Geometry check sheet. Reference: the model listing, model coordinates, mm. A direction names the side the tool comes from. Round coordinates to 2 decimals unless told otherwise and drop trailing zeros. Write each loop counter-clockwise with the first axis right and the second up, starting at its lowest first coordinate (ties: lowest second). Pieces come first, ordered by that corner, then holes.
Item 1: Draft check along Z on faces 4 (the face through (0, -11, -14)), 5 (the face through (23, 13, 3)), 6 (the face through (0.1, 14.5, 4.15)), 7 (the face through (-26, -8, -2)). Enter one of: pulls with the +Z half, pulls with the -Z half, needs draft (parallel to the pull), parting line crosses it, or undercut.
Item 2: Cross-section at A-A (z = -9). Enter the section's corners in (x, y) (3 decimals), then the cut area to 3 significant figures.
Item 3: Cross-section at C-C (x = 18). Enter the section's corners in (y, z).
Item 4: Access from +Z, -Z, +X, -X, +Y, -Y to the whole of each face (thin tool, end or side, straight path). Record for faces 1 (the face through (0.1, 14.5, 1.85)), 2 (the face through (0, -9, -9)), 3 (the face through (0, 11.6, 3)).
Item 5: Cross-section at B-B (y = -12). Enter the section's corners in (x, z) (3 decimals), then the cut area to 3 significant figures.
Item 6: Scan lines: probe 1 along Z at (x, y) = (19, -10.55) (3 decimals); probe 2 along Y at (x, z) = (-15, 1.5); probe 3 along Y at (x, z) = (-0.5, 1.5). Record each from-to range of solid material in increasing order.
Item 7: Cross-section at D-D (y = 2.75). Enter the section's corners in (x, z).
Item 8: Depth check by flat-ended pin: P1, Ø4, axis at y = 2.5, z = -2.5, coming from the +X side; P2, Ø6, axis at x = 6, y = 8.5, coming from the -Z side; P3, Ø1.8, axis at x = -15.5, z = 3, coming from the +Y side; P4, Ø1.5, axis at x = -0.5, z = 1.5, coming from the -Y side. Enter the tip coordinate at first touch or a pass-through.
from build123d import *

# Parameters (mm, degrees)
SKETCH_W        = 52
SKETCH_H        = 30
PAD_DEPTH       = 6
SKETCH001_R     = 6.15
POCKET_DEPTH    = 6
SKETCH002_W     = 30
SKETCH002_H     = 2.3
POCKET001_DEPTH = 2
SKETCH003_W     = 52
SKETCH003_H     = 2.3
POCKET002_DEPTH = 2
SKETCH004_W     = 30
SKETCH004_H     = 2.3
POCKET003_DEPTH = 2
SKETCH005_W     = 52
SKETCH005_H     = 6
PAD001_DEPTH    = 14
SKETCH006_W     = 19.5
SKETCH006_H     = 3.75
POCKET004_DEPTH = 26
CHAMFER_SIZE    = 4
SKETCH007_W     = 45
SKETCH007_H     = 2
PAD002_DEPTH    = 6
SKETCH008_R     = 1.875
POCKET005_DEPTH = 6


with BuildPart() as part:
    # Sketch → Pad (new body)
    with BuildSketch(Plane.XY):
        Rectangle(SKETCH_W, SKETCH_H)
    extrude(amount=PAD_DEPTH)

    # Sketch001 (on Face6 of Pad) → Pocket (cut)
    with BuildSketch(Plane.XY.offset(6)):
        with Locations((-16, 6)):
            Circle(SKETCH001_R)
        with Locations((0, 6)):
            Circle(SKETCH001_R)
        with Locations((16, 6)):
            Circle(SKETCH001_R)
    extrude(amount=-POCKET_DEPTH, mode=Mode.SUBTRACT)

    # Sketch002 (on Face3 of Pocket) → Pocket001 (cut)
    with BuildSketch(Plane.YZ.offset(26)):
        with Locations((0, 3)):
            Rectangle(SKETCH002_W, SKETCH002_H)
    extrude(amount=-POCKET001_DEPTH, mode=Mode.SUBTRACT)

    # Sketch003 (on Face1 of Pocket001) → Pocket002 (cut)
    with BuildSketch(Plane(origin=(0, 15, 0), x_dir=(-1, 0, 0), z_dir=(0, 1, 0))):
        with Locations((0, 3)):
            Rectangle(SKETCH003_W, SKETCH003_H)
    extrude(amount=-POCKET002_DEPTH, mode=Mode.SUBTRACT)

    # Sketch004 (on Face6 of Pocket002) → Pocket003 (cut)
    with BuildSketch(Plane(origin=(-26, 0, 0), x_dir=(0, -1, 0), z_dir=(-1, 0, 0))):
        with Locations((0, 3)):
            Rectangle(SKETCH004_W, SKETCH004_H)
    extrude(amount=-POCKET003_DEPTH, mode=Mode.SUBTRACT)

    # Sketch005 (on Face2 of Pocket003) → Pad001 (join)
    with BuildSketch(Plane(origin=(0, 0, 0), x_dir=(1, 0, 0), z_dir=(0, 0, -1))):
        with Locations((0, 12)):
            Rectangle(SKETCH005_W, SKETCH005_H)
    extrude(amount=PAD001_DEPTH)

    # Sketch006 (on Face19 of Pad001) → Pocket004 (cut)
    with BuildSketch(Plane.XY.offset(6)):
        with Locations((1.25, -13.125)):
            Rectangle(SKETCH006_W, SKETCH006_H)
    extrude(amount=-POCKET004_DEPTH, mode=Mode.SUBTRACT)

    # Chamfer
    chamfer_edges = [part.edges().sort_by_distance(p)[0] for p in [
        (0, -9, 0),
    ]]
    chamfer(chamfer_edges, length=CHAMFER_SIZE)

    # Sketch007 (on Face19 of Chamfer) → Pad002 (join)
    with BuildSketch(Plane.XY.offset(6)):
        with Locations((0, -0.4)):
            Rectangle(SKETCH007_W, SKETCH007_H)
        with Locations((0, 12.6)):
            Rectangle(SKETCH007_W, SKETCH007_H)
    extrude(amount=-PAD002_DEPTH)

    # Sketch008 (on Face16 of Pad002) → Pocket005 (cut)
    with BuildSketch(Plane(origin=(0, -9, 0), x_dir=(-1, 0, 0), z_dir=(0, 1, 0))):
        with Locations((-19, -9)):
            Circle(SKETCH008_R)
        with Locations((19, -9)):
            Circle(SKETCH008_R)
    extrude(amount=-POCKET005_DEPTH, mode=Mode.SUBTRACT)


solid = part.part
Resolved:
1. face 4: pulls with the -Z half
1. face 5: undercut
1. face 6: undercut
1. face 7: needs draft
2. outline: (-26, -15) - (-20.875, -15) - (-20.875, -9) - (-26, -9) - close; (-17.125, -15) - (-8.5, -15) - (-8.5, -11.25) - (11, -11.25) - (11, -15) - (17.125, -15) - (17.125, -9) - (-17.125, -9) - close; (20.875, -15) - (26, -15) - (26, -9) - (20.875, -9) - close
2. area: 194 mm2
3. outline: (-15, -14) - (-9, -14) - (-9, -10.59) - (-15, -10.59) - close; (-15, -7.41) - (-9, -7.41) - (-9, -4) - (-5, 0) - (0.6, 0) - (0.6, 6) - (-15, 6) - close; (11.6, 0) - (15, 0) - (15, 1.85) - (13.6, 1.85) - (13.6, 4.15) - (15, 4.15) - (15, 6) - (11.6, 6) - close
4. face 1: +Y
4. face 2: -Z, +X, -X, +Y
4. face 3: +Z, -Z
5. outline: (-26, -14) - (-8.5, -14) - (-8.5, 6) - (-26, 6) - (-26, 4.15) - (-24, 4.15) - (-24, 1.85) - (-26, 1.85) - close; (11, -14) - (26, -14) - (26, 1.85) - (24, 1.85) - (24, 4.15) - (26, 4.15) - (26, 6) - (11, 6) - close; hole circle Ø3.75 at (-19, -9); hole circle Ø3.75 at (19, -9)
5. area: 619 mm2
6. probe 1: z = -14 to -10.875, -7.125 to 6
6. probe 2: y = -15 to 0.6, 11.6 to 15
6. probe 3: y = -11.25 to 0.6, 11.6 to 15
7. outline: (-26, 0) - (-21.22, 0) - (-21.22, 6) - (-26, 6) - (-26, 4.15) - (-24, 4.15) - (-24, 1.85) - (-26, 1.85) - close; (-10.78, 0) - (-5.22, 0) - (-5.22, 6) - (-10.78, 6) - close; (5.22, 0) - (10.78, 0) - (10.78, 6) - (5.22, 6) - close; (21.22, 0) - (26, 0) - (26, 1.85) - (24, 1.85) - (24, 4.15) - (26, 4.15) - (26, 6) - (21.22, 6) - close
8. P1: passes through
8. P2: stops at z = 0
8. P3: stops at y = 13.6
8. P4: stops at y = -11.25
